CAD build for the part. Positions are in the model's coordinates, mm. Coordinates: 2 decimals unless noted, no trailing zeros. Write each loop counter-clockwise with the first axis right and the second up, starting at its lowest first coordinate (ties: lowest second). Pieces come first, ordered by that corner, then holes. Notation, with made-up numbers: (-32.75, 42.5) - (13.25, 42.5) arc R11 cw to (13.25, 61.5) - close; hole circle Ø6 at (66.5, -26). An arc over 180 degrees is marked (long way). Answer in a Markdown table with one row per item. Add a question column.
Q1. Two-plate mould, pull along Y, no slides. Class faces 1 (the flat face through (10, 10, 0)), 2 (the flat face through (-20, 0, 0)), 3 (the cylindrical face through (-12.4, 18.2, -1.5)): +Y half, -Y half, draft (parallel to the pull), parting line (faces both ways), or undercut.
Q2. Band-saw the part on B-B (x = 10). List the corners of the cut face in (y, z), and give its area (3 significant figures).
Q3. Band-saw the part on C-C (y = 20). List the corners of the cut face in (x, z), and give its area (3 significant figures).
Q4. Band-saw the part on A-A (y = -20). List the corners of the cut face in (x, z), and give its area (3 significant figures).
Q5. Band-saw the part on D-D (z = 0.7). List the corners of the cut face in (x, y).
Q6. Drill centre lines: line 1 along Y through (x, z) = (-10, -1.5); line 2 along Y through (x, z) = (-8, -0.85); line 3 along Y through (x, z) = (11, -1.5). Where is each one in solid material? Low to high. Write a range as from..to.
```python
from build123d import *

# Parameters (mm, degrees)
BOSS_EXTRUDE1_DEPTH = 1.708
SKETCH2_R           = 3
CUT_EXTRUDE1_DEPTH  = 4.416
CHAMFER1_SIZE       = 3


with BuildPart() as part:
    # Sketch1 → Boss-Extrude1 (new body, symmetric)
    with BuildSketch(Plane.XY):
        Polygon((-20, -30), (-20, 30), (0, 30), (20, -10), (20, -30), align=None)
    extrude(amount=BOSS_EXTRUDE1_DEPTH, both=True)

    # Sketch2 → Cut-Extrude1 (cut, through all)
    with BuildSketch(Plane.XY.offset(1.708)):
        with Locations((-10, 20)):
            Circle(SKETCH2_R)
        with Locations((-10, -20)):
            Circle(SKETCH2_R)
        with Locations((10, -20)):
            Circle(SKETCH2_R)
    extrude(amount=-CUT_EXTRUDE1_DEPTH, mode=Mode.SUBTRACT)

    # Chamfer1
    chamfer1_edges = [part.edges().sort_by_distance(p)[0] for p in [
        (-13, 20, 1.708),
        (-13, -20, 1.708),
        (7, -20, 1.708),
    ]]
    chamfer(chamfer1_edges, length=CHAMFER1_SIZE)


solid = part.part
```
Checked values:
| question | item | result |
|---|---|---|
| 1 | face 1 | +Y half |
| 1 | face 2 | draft |
| 1 | face 3 | undercut |
| 2 | outline | (-30, -1.71) - (-23, -1.71) - (-23, -1.29) - (-26, 1.71) - (-30, 1.71) - close; (-17, -1.71) - (10, -1.71) - (10, 1.71) - (-14, 1.71) - (-17, -1.29) - close |
| 2 | area | 107 mm² |
| 3 | outline | (-20, -1.71) - (-13, -1.71) - (-13, -1.29) - (-16, 1.71) - (-20, 1.71) - close; (-7, -1.71) - (5, -1.71) - (5, 1.71) - (-4, 1.71) - (-7, -1.29) - close |
| 3 | area | 55.9 mm² |
| 4 | outline | (-20, -1.71) - (-13, -1.71) - (-13, -1.29) - (-16, 1.71) - (-20, 1.71) - close; (-7, -1.71) - (7, -1.71) - (7, -1.29) - (4, 1.71) - (-4, 1.71) - (-7, -1.29) - close; (13, -1.71) - (20, -1.71) - (20, 1.71) - (16, 1.71) - (13, -1.29) - close |
| 4 | area | 77.6 mm² |
| 5 | outline | (-20, -30) - (20, -30) - (20, -10) - (0, 30) - (-20, 30) - close; hole circle Ø9.98 at (-10, -20); hole circle Ø9.98 at (-10, 20); hole circle Ø9.98 at (10, -20) |
| 6 | line 1 | y = -30..-23, -17..17, 23..30 |
| 6 | line 2 | y = -30..-22.8, -17.2..17.2, 22.8..30 |
| 6 | line 3 | y = -30..-22.83, -17.17..8 |
